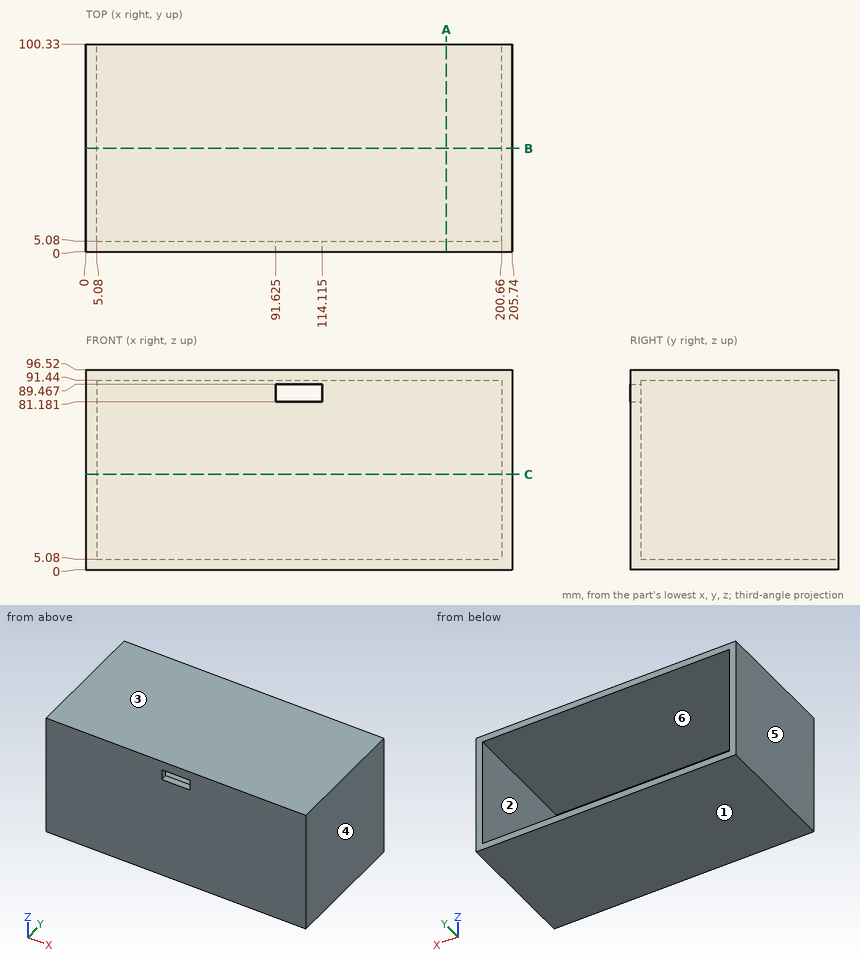
Here's the drawing with two shaded views (mm, measured from the low corner). I have some questions. A direction names the side the tool comes from. Coordinates: 2 decimals unless noted, no trailing zeros. Write each loop counter-clockwise with the first axis right and the second up, starting at its lowest first coordinate (ties: lowest second). Pieces come first, ordered by that corner, then holes. Notation, with made-up numbers: (48.5, 79.5) -> (61.5, 79.5) arc R25 cw to (61.5, 104.5) -> close; hole circle Ø9 at (0.5, -13.5). An arc over 180 degrees is marked (long way). One line per question, with ' | ' between items. Start each with the question number.
1. Please list where these lines run through material, in increasing order: line 1 along X through (y, z) = (51, 30); line 2 along Z through (x, y) = (155, 79.5); line 3 along Y through (x, z) = (23, 69.5).
2. Will this pin go through, and if not, where does the flat tip stop? P1, Ø4, axis at x = 165, z = 78, coming from the +Y side.
3. If we section it at C-C (z = 46): Please give me the cut outline in (x, y), and give its area (3 significant figures).
4. For the marked faces 5 and 6, which set-ups out of +Z, -Z, +X, -X, +Y, -Y let a thin tool reach every point of the face, with its end or its side?
5. Thinking about a two-plate mould opening in Z: for the marked faces 1, 2, 3 and 4, which applies, pulls with the +Z half, pulls with the -Z half, needs draft (parallel to the pull), parting line crosses it, or undercut?
6. If we section it at A-A (x = 174): Please give me the cut outline in (y, z).
7. If we section it at B-B (y = 50): Please give me the cut outline in (x, z).
Return value:
1) line 1: x = 0 to 5.08, 200.66 to 205.74 | line 2: z = 0 to 5.08, 91.44 to 96.52 | line 3: y = 0 to 5.08
2) P1: stops at y = 5.08
3) outline: (0, 0) -> (205.74, 0) -> (205.74, 100.33) -> (200.66, 100.33) -> (200.66, 5.08) -> (5.08, 5.08) -> (5.08, 100.33) -> (0, 100.33) -> close | area: 2,010 mm²
4) face 5: +Z, -Z, -X, +Y, -Y | face 6: +Y
5) face 1: pulls with the -Z half | face 2: undercut | face 3: pulls with the +Z half | face 4: needs draft
6) outline: (0, 0) -> (100.33, 0) -> (100.33, 5.08) -> (5.08, 5.08) -> (5.08, 91.44) -> (100.33, 91.44) -> (100.33, 96.52) -> (0, 96.52) -> close
7) outline: (0, 0) -> (205.74, 0) -> (205.74, 96.52) -> (0, 96.52) -> close; hole (5.08, 5.08) -> (200.66, 5.08) -> (200.66, 91.44) -> (5.08, 91.44) -> close
